The listing builds one solid part. Answer for the finished solid, in the listing's coordinates (mm). Face numbers are marked on the shaded views. A direction names the side the tool comes from. Round coordinates to 2 decimals unless told otherwise and drop trailing zeros. Loops run counter-clockwise (first coordinate to the right, second up) from the corner with the lowest first, then second, coordinate; pieces in that order, holes last. Notation, with made-up numbers: M 19.25,-23 L 60.25,-23 A25 ccw 60.25,-6 Z; hole C 20.5,34.25 d1. An arc over 180 degrees is marked long. Put each result on its own line as item: value. Start each with the question number.
(1) Section C-C, the plane y = 14 is taken. Determine the outline of the cut face in (x, z), then the cut area to 3 significant figures.
(2) Section D-D, the plane z = 20 is taken. Determine the outline of the cut face in (x, y), then the cut area to 3 significant figures.
(3) Flat-ended cylindrical pins translate along their axes: P1, Ø13, axis at y = -1.5, z = 17.5, coming from the +X side; P2, Ø12, axis at y = -13, z = 24.5, coming from the +X side; P3, Ø5, axis at x = 0, z = 13, coming from the +Y side. Find the tip coordinate at first contact, or state that the pin passes through.
(4) Which of the six approach directions +Z, -Z, +X, -X, +Y, -Y give full straight-line access (tool end or side, diameter ignored) to the marked faces 1, 2 and 3?
(5) Straight lines are drawn through the part: line 1 (Y direction, x = 0, z = 1.9); line 2 (X direction, y = 2.5, z = 15); line 3 (Z direction, x = 0, y = 0). For each, find the intervals that lie inside material, in ascending order.
(6) Section B-B, the plane z = 14.5 is taken. Determine the outline of the cut face in (x, y), then the cut area to 3 significant figures.
(7) Section A-A, the plane x = 0 is taken. Determine the outline of the cut face in (y, z), then the cut area to 3 significant figures.
```python
from build123d import *

# Parameters (mm, degrees)
F0_W      = 20
F0_H      = 40
F1_DEPTH  = 4
F2_W      = 8
F2_H      = 16
F3_DEPTH  = 25
F5_DEPTH  = 25
F6_R      = 5
F7_R      = 2
F8_R      = 2
F9_DEPTH  = 25
F10_R     = 1.4745216426
F11_DEPTH = 5
F13_DEPTH = 2


with BuildPart() as f1:
    # F0 (on Top) → F1 (new body)
    with BuildSketch(Plane.XY):
        Rectangle(F0_W, F0_H)
    extrude(amount=F1_DEPTH)

    # F2 (on face) → F3 (join)
    with BuildSketch(Plane.XY.offset(4)):
        Rectangle(F2_W, F2_H)
    extrude(amount=F3_DEPTH)

    # F4 (on face) → F5 (cut)
    with BuildSketch(Plane.YZ.offset(4)):
        with BuildLine():
            Line((-8, 29), (-8, 26.6885775404))
            ThreePointArc((-8, 26.6885775404), (-4.1636124275, 28.4105631935), (0, 29))
            Line((0, 29), (-8, 29))
        make_face()
        with BuildLine():
            ThreePointArc((0, 29), (4.1636124275, 28.4105631935), (8, 26.6885775404))
            Line((8, 26.6885775405), (8, 29))
            Line((8, 29), (0, 29))
        make_face()
    extrude(amount=-F5_DEPTH, mode=Mode.SUBTRACT)

    # F6
    f6_edges = [f1.edges().sort_by_distance(p)[0] for p in [
        (-10, 20, 2),
        (-10, -20, 2),
        (10, -20, 2),
        (10, 20, 2),
    ]]
    fillet(f6_edges, radius=F6_R)

    # F7
    f7_edges = [f1.edges().sort_by_distance(p)[0] for p in [
        (10, 0, 4),
        (8.535534, -18.535534, 4),
        (8.535534, 18.535534, 4),
        (0, -20, 4),
        (0, 20, 4),
        (-8.535534, -18.535534, 4),
        (-8.535534, 18.535534, 4),
        (-10, 0, 4),
        (4, 0, 4),
        (0, 8, 4),
        (-4, 0, 4),
        (0, -8, 4),
        (4, -8, 15.344289),
        (4, 0, 29),
        (4, 8, 15.344289),
        (-4, 8, 15.344289),
        (-4, 0, 29),
        (-4, -8, 15.344289),
    ]]
    fillet(f7_edges, radius=F7_R)

    # F8 (on face) → F9 (cut)
    with BuildSketch(Plane(origin=(-4, 0, 0), x_dir=(0, -1, 0), z_dir=(-1, 0, 0))):
        with Locations((0, 20)):
            Circle(F8_R)
    extrude(amount=-F9_DEPTH, mode=Mode.SUBTRACT)

    # F10 (on face) → F11 (cut)
    with BuildSketch(Plane.XY.offset(4)):
        with Locations((0, 14.610607177)):
            Circle(F10_R)
        with Locations((0, -14.610607177)):
            Circle(F10_R)
    extrude(amount=-F11_DEPTH, mode=Mode.SUBTRACT)

    # F12 (on face) → F13 (cut)
    with BuildSketch(Plane.YZ.offset(4)):
        Polygon((3, 21.7320508076), (0, 23.4641016151), (-3, 21.7320508076), (-3, 18.2679491924), (0, 16.5358983849), (3, 18.2679491924), align=None)
    extrude(amount=-F13_DEPTH, mode=Mode.SUBTRACT)


solid = f1.part
```
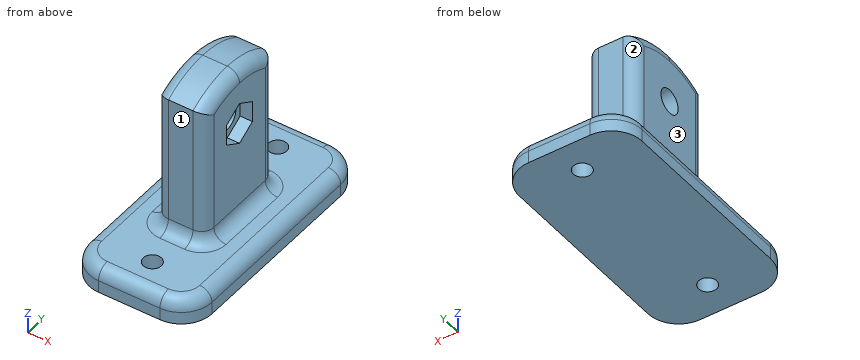
Recorded:
1. outline: M -10,0 L -1.34,0 L -1.34,4 L -8,4 A2 ccw -10,2 Z; M 1.34,0 L 10,0 L 10,2 A2 ccw 8,4 L 1.34,4 Z
1. area: 67.5 mm²
2. outline: M -4,-6 A2 ccw -2,-8 L 2,-8 A2 ccw 4,-6 L 4,-3 L 2,-3 L 2,-2 L -4,-2 Z; M -4,2 L 2,2 L 2,3 L 4,3 L 4,6 A2 ccw 2,8 L -2,8 A2 ccw -4,6 Z
2. area: 88.6 mm²
3. P1: stops at x = 4
3. P2: stops at x = 3.73
3. P3: stops at y = 8
4. face 1: +Z, +X, -X, -Y
4. face 2: +Z, -X, +Y
4. face 3: +Z, -X, +Y, -Y
5. line 1: y = -20 to -16.09, -13.14 to 13.14, 16.09 to 20
5. line 2: x = -4 to 4
5. line 3: z = 0 to 18, 22 to 29
6. outline: M -4,-6 A2 ccw -2,-8 L 2,-8 A2 ccw 4,-6 L 4,6 A2 ccw 2,8 L -2,8 A2 ccw -4,6 Z
6. area: 125 mm²
7. outline: M -20,0 L -16.09,0 L -16.09,4 L -18,4 A2 ccw -20,2 Z; M -13.14,0 L 13.14,0 L 13.14,4 L 10,4 A2 cw 8,6 L 8,26.69 A15 ccw -8,26.69 L -8,6 A2 cw -10,4 L -13.14,4 Z; M 16.09,0 L 20,0 L 20,2 A2 ccw 18,4 L 16.09,4 Z; hole C 0,20 d4
7. area: 512 mm²
